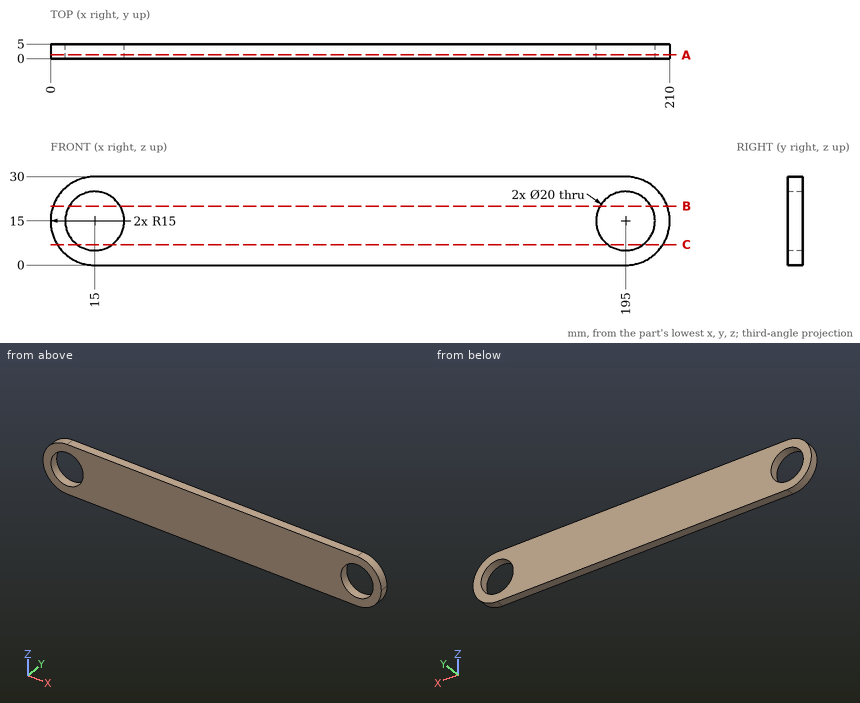
Source: three-view drawing plus pictorial views. Frame: mm from the lowest corner of the part. Round coordinates to 2 decimals unless told otherwise and drop trailing zeros. Loops run counter-clockwise (first coordinate to the right, second up) from the corner with the lowest first, then second, coordinate; pieces in that order, holes last. Notation, with made-up numbers: M -3.5,70 L 25.5,70 A14 cw 25.5,87 Z; hole C 55.25,38 d4. An arc over 180 degrees is marked long. Put each result on its own line as item: value.
(1) Section B-B, the plane z = 20. Return loops of the section in (x, y).
Solutions:
outline: M 0.86,0 L 6.34,0 L 6.34,5 L 0.86,5 Z; M 23.66,0 L 186.34,0 L 186.34,5 L 23.66,5 Z; M 203.66,0 L 209.14,0 L 209.14,5 L 203.66,5 Z
(2) Ray query, line 1 (Z direction, x = 15, y = 3.65); line 2 (X direction, y = 3.35, z = 12.5); line 3 (X direction, y = 2.45, z = 10). Return the intervals inside material, ascending. Write a range as [from, to].
Solutions:
line 1: [0, 5], [25, 30]
line 2: [0.21, 5.32], [24.68, 185.32], [204.68, 209.79]
line 3: [0.86, 6.34], [23.66, 186.34], [203.66, 209.14]
(3) Section A-A, the plane y = 1.3. Return loops of the section in (x, z).
Solutions:
outline: M 15,0 L 195,0 A15 ccw 210,15 A15 ccw 195,30 L 15,30 A15 ccw Z; hole C 15,15 d20; hole C 195,15 d20
(4) Section C-C, the plane z = 7. Return loops of the section in (x, y).
Solutions:
outline: M 2.31,0 L 9,0 L 9,5 L 2.31,5 Z; M 21,0 L 189,0 L 189,5 L 21,5 Z; M 201,0 L 207.69,0 L 207.69,5 L 201,5 Z
(5) First-contact query: pin 1 (2 mm diameter, centred on y = 1, z = 13, fed in from +X); pin 2 (2 mm diameter, centred on y = 3, z = 20, fed in from +X). Flat tips, straight axial feed; report the tip coordinate or a pass-through.
Solutions:
pin 1: x = 209.97
pin 2: x = 209.46
